Input: part model. Units: mm. Frame: model coordinates. A direction names the side the tool comes from. Coordinates: 2 decimals unless noted, no trailing zeros. Order: outer loops, then holes, each group sorted by start corner. A loop starts at its lowest first (then second) coordinate and runs counter-clockwise, first axis right, second up. Notation, with made-up numbers: M 70,82.5 L 127,82.5 A18 cw 127,106.5 Z; hole C 48,-20.75 d2. An arc over 180 degrees is marked long. One line per item, written item: value.
```python
from build123d import *

# Parameters (mm, degrees)
BASPROSKE_W        = 6
BASPROSKE_H        = 10
TOOTHCUT_DEPTH     = 16.362291496
TEETHCUTS_COUNT    = 18
TEETHCUTS_ANGLE    = 340
CUT_EXTRUDE1_DEPTH = 16.289512146


with BuildPart() as part:
    # BasProSke → Base-Revolve (revolve)
    with BuildSketch(Plane(origin=(0, 0, 0), x_dir=(1, 0, 0), z_dir=(0, 1, 0)), mode=Mode.PRIVATE) as base_revolve_sk:
        with Locations((3, 5)):
            Rectangle(BASPROSKE_W, BASPROSKE_H)
    revolve(base_revolve_sk.sketch.rotate(Axis((-10, 0, 0), (1, 0, 0)), 180), axis=Axis((-10, 0, 0), (1, 0, 0)))

    # TooCutSke → ToothCut (cut, through all)
    with BuildSketch(Plane(origin=(0, 0, 0), x_dir=(0, 0, -1), z_dir=(1, 0, 0))):
        with BuildLine():
            ThreePointArc((0.510641536, 7.732156635), (0, 7.749), (-0.510641536, 7.732156635))
            ThreePointArc((-0.510641536, 7.732156635), (-0.82619259, 8.907320741), (-1.515208602, 9.910236529))
            ThreePointArc((-1.515208602, 9.910236529), (0, 10.0254), (1.515208602, 9.910236529))
            ThreePointArc((1.515208602, 9.910236529), (0.82619259, 8.907320741), (0.510641536, 7.732156635))
        make_face()
    toothcut = extrude(amount=TOOTHCUT_DEPTH, mode=Mode.SUBTRACT)

    # TeethCuts: ToothCut ×18 about axis
    teethcuts_axis = Axis((-10, 0, 0), (1, 0, 0))
    for i in range(1, TEETHCUTS_COUNT):
        add(toothcut.rotate(teethcuts_axis, i * TEETHCUTS_ANGLE / (TEETHCUTS_COUNT - 1)), mode=Mode.SUBTRACT)

    # Sketch1 → Cut-Extrude1 (cut, through all)
    with BuildSketch(Plane(origin=(6, 0, 0), x_dir=(0, 0, -1), z_dir=(1, 0, 0))):
        with BuildLine():
            Line((2.277471185, 1.875), (2.277471185, -1.875))
            ThreePointArc((2.277471185, -1.875), (-2.95, 0), (2.277471185, 1.875))
        make_face()
    extrude(amount=-CUT_EXTRUDE1_DEPTH, mode=Mode.SUBTRACT)


solid = part.part
```
(1) Ray query, line 1 (Z direction, x = 4.4, y = 0); line 2 (Y direction, x = 2.2, z = 8.5); line 3 (Y direction, x = 2.6, z = 0). Return the intervals inside material, ascending. Write a range as from..to.
Data:
line 1: z = -10..-2.28, 2.95..10
line 2: y = -3.75..-2.28, -0.82..0.82, 2.28..3.75
line 3: y = -7.75..-2.95, 2.95..7.75
(2) First-contact query: pin 1 (2 mm diameter, centred on x = 2, z = 4, fed in from +Y). Flat tip, straight axial feed; report the tip coordinate or a pass-through.
Data:
pin 1: stops at y = 8.78
(3) Draft query along Y for faces 1 (the cylindrical face through (2.958, -8.878, -0.813)), 2 (the cylindrical face through (2.958, -3.881, -6.707)), 3 (the cylindrical face through (2.96, 5.14, -7.28)), 4 (the cylindrical face through (2.958, 8.878, 0.813)). Return one class per face: released by +Y, released by -Y, zero draft, split by the parting line, or undercut.
Data:
face 1: released by -Y
face 2: undercut
face 3: undercut
face 4: released by +Y
(4) Access query for faces 5 (the cylindrical face through (2.96, -5.14, 7.28)), 6 (the flat face through (3, 0, -2.277)), 7 (the flat face through (0, 2.1, 2.4)), 8 (the cylindrical face through (2.958, 8.089, -3.824)), 9 (the cylindrical face through (2.96, 2.34, -8.6)). Directions: +Z, -Z, +X, -X, +Y, -Y. A direction counts if a zero-diameter tool reaches every point of the face in a straight line with its end or side. Return the directions, or none.
Data:
face 5: +Z, +X, -X
face 6: +X, -X
face 7: +Z, -Z, -X, +Y, -Y
face 8: +X, -X, +Y
face 9: -Z, +X, -X
(5) Cut plane A-A on y = 0. Output: boundary loops of the cut face in (x, z).
Data:
outline: M 0,-10 L 6,-10 L 6,-2.28 L 0,-2.28 Z; M 0,2.95 L 6,2.95 L 6,10 L 0,10 Z
(6) Cut plane B-B on z = 0. Output: boundary loops of the cut face in (x, y).
Data:
outline: M 0,-7.75 L 6,-7.75 L 6,-2.95 L 0,-2.95 Z; M 0,2.95 L 6,2.95 L 6,7.75 L 0,7.75 Z
